Could you check a few things on this model? Use its own coordinates, in mm. A direction names the side the tool comes from. Give positions to 0.01 mm unless a question says otherwise; leave off trailing zeros. Loops run counter-clockwise (first coordinate to the right, second up) from the corner with the lowest first, then second, coordinate; pieces in that order, holes last. Notation, with made-up numbers: M 72,42 L 82,42 A17 cw 82,49 Z; hole C -10.5,61.5 d11. An arc over 180 degrees is marked long. Answer in a Markdown table with one row per item. Add a question column.
1. If we section it at C-C on z = 10: List the corners of the cut face in (x, y) for me.
2. If we section it at D-D on y = -9: List the corners of the cut face in (x, z) for me (3 decimals), then the cut area to 3 significant figures.
3. I'm going to push flat-ended pins straight in: pin 1 Ø3.5 at (y, z) = (7, 10) entering from +X; pin 2 Ø1 at (y, z) = (-5, 1) entering from -X; pin 3 Ø1.8 at (x, z) = (-8.5, 10.5) entering from -Y; pin 4 Ø5 at (x, y) = (-8.5, -8.5) entering from +Z. Where does each tip first touch, or does it pass through?
4. Which directions (+Z, -Z, +X, -X, +Y, -Y) give clear straight access to the entire face, cutting with the end or side of a thin tool? Please do faces 4 (the flat face through (-6, 6, 8)), 5 (the cylindrical face through (-6.57, 6.52, 2.45)), 6 (the cylindrical face through (-9.993, 6.599, 7.752)).
5. I need wall thicknesses on line 1 along Y through (x, z) = (0, 0.5) (3 decimals); line 2 along Z through (x, y) = (-7.05, 6.5); line 3 along Z through (x, y) = (-3.75, 0). Which ranges of each line are inside material? Lowest first, please. Write a range as from..to.
6. If we section it at A-A on y = 6.5: List the corners of the cut face in (x, z) for me, then the cut area to 3 significant figures.
7. If we section it at B-B on x = 0: List the corners of the cut face in (y, z) for me (3 decimals), then the cut area to 3 significant figures.
8. Thinking about a two-plate mould opening in Y: for faces 1 (the cylindrical face through (-0.179, -7.637, 1.014)), 2 (the flat face through (-4.5, -6, 1)), 3 (the cylindrical face through (-4.95, 1.57, 1.06)), which applies, released by +Y, released by -Y, zero draft, split by the parting line, or undercut?
```python
from build123d import *

# Parameters (mm, degrees)
SKETCH1_W           = 9
SKETCH1_H           = 22
BOSS_EXTRUDE1_DEPTH = 2
SKETCH2_R           = 2.5
SKETCH2_R_2         = 1.375
CUT_EXTRUDE1_DEPTH  = 2
SKETCH3_W           = 2
SKETCH3_H           = 9
BOSS_EXTRUDE2_DEPTH = 5
SKETCH5_W           = 2.5
SKETCH5_H           = 9
BOSS_EXTRUDE4_DEPTH = 12.5
SKETCH6_R           = 1.75
CUT_EXTRUDE2_DEPTH  = 2.5
SKETCH7_R           = 2.25
BOSS_EXTRUDE5_DEPTH = 1
SKETCH8_R           = 1.75
CUT_EXTRUDE3_DEPTH  = 1
SKETCH9_R           = 2.25
BOSS_EXTRUDE6_DEPTH = 1
SKETCH10_R          = 1.75
CUT_EXTRUDE4_DEPTH  = 1
FILLET1_R           = 1.5
FILLET2_R           = 1.5
SKETCH11_W          = 9
SKETCH11_H          = 2
BOSS_EXTRUDE7_DEPTH = 1.5


with BuildPart() as part:
    # Sketch1 → Boss-Extrude1 (new body)
    with BuildSketch(Plane.XY):
        Rectangle(SKETCH1_W, SKETCH1_H)
    extrude(amount=BOSS_EXTRUDE1_DEPTH)

    # Sketch2 → Cut-Extrude1 (cut)
    with BuildSketch(Plane.XY.offset(2)):
        with Locations((0, 6.5)):
            Circle(SKETCH2_R)
        with Locations((0, -9)):
            Circle(SKETCH2_R_2)
    extrude(amount=-CUT_EXTRUDE1_DEPTH, mode=Mode.SUBTRACT)

    # Sketch3 → Boss-Extrude2 (add)
    with BuildSketch(Plane.ZY.offset(4.5)):
        with Locations((1, 6.5)):
            Rectangle(SKETCH3_W, SKETCH3_H)
    extrude(amount=BOSS_EXTRUDE2_DEPTH)

    # Sketch5 → Boss-Extrude4 (add)
    with BuildSketch(Plane.XY.offset(2)):
        with Locations((-8.25, 6.5)):
            Rectangle(SKETCH5_W, SKETCH5_H)
    extrude(amount=BOSS_EXTRUDE4_DEPTH)

    # Sketch6 → Cut-Extrude2 (cut)
    with BuildSketch(Plane(origin=(-7, 0, 0), x_dir=(0, 0, -1), z_dir=(1, 0, 0))):
        with Locations((-10, 6.5)):
            Circle(SKETCH6_R)
    extrude(amount=-CUT_EXTRUDE2_DEPTH, mode=Mode.SUBTRACT)

    # Sketch7 → Boss-Extrude5 (add)
    with BuildSketch(Plane(origin=(-7, 0, 0), x_dir=(0, 0, -1), z_dir=(1, 0, 0))):
        with Locations((-10, 6.5)):
            Circle(SKETCH7_R)
    extrude(amount=BOSS_EXTRUDE5_DEPTH)

    # Sketch8 → Cut-Extrude3 (cut)
    with BuildSketch(Plane(origin=(-6, 0, 0), x_dir=(0, 0, -1), z_dir=(1, 0, 0))):
        with Locations((-10, 6.5)):
            Circle(SKETCH8_R)
    extrude(amount=-CUT_EXTRUDE3_DEPTH, mode=Mode.SUBTRACT)

    # Sketch9 → Boss-Extrude6 (add)
    with BuildSketch(Plane.ZY.offset(9.5)):
        with Locations((10, 6.5)):
            Circle(SKETCH9_R)
    extrude(amount=BOSS_EXTRUDE6_DEPTH)

    # Sketch10 → Cut-Extrude4 (cut)
    with BuildSketch(Plane.ZY.offset(10.5)):
        with Locations((10, 6.5)):
            Circle(SKETCH10_R)
    extrude(amount=-CUT_EXTRUDE4_DEPTH, mode=Mode.SUBTRACT)

    # Fillet1
    fillet1_edges = [part.edges().sort_by_distance(p)[0] for p in [
        (-7, 6.5, 2),
    ]]
    fillet(fillet1_edges, radius=FILLET1_R)

    # Fillet2
    fillet2_edges = [part.edges().sort_by_distance(p)[0] for p in [
        (-4.5, 2, 1),
    ]]
    fillet(fillet2_edges, radius=FILLET2_R)

    # Sketch11 → Boss-Extrude7 (add)
    with BuildSketch(Plane.XZ.offset(11)):
        with Locations((0, 1)):
            Rectangle(SKETCH11_W, SKETCH11_H)
    extrude(amount=BOSS_EXTRUDE7_DEPTH)


solid = part.part
```
Results:
| question | item | result |
|---|---|---|
| 1 | outline | M -10.5,4.25 L -9.5,4.25 L -9.5,2 L -7,2 L -7,4.25 L -6,4.25 L -6,4.75 L -10.5,4.75 Z; M -10.5,8.25 L -6,8.25 L -6,8.75 L -7,8.75 L -7,11 L -9.5,11 L -9.5,8.75 L -10.5,8.75 Z |
| 2 | outline | M -4.5,0 L -1.375,0 L -1.375,2 L -4.5,2 Z; M 1.375,0 L 4.5,0 L 4.5,2 L 1.375,2 Z |
| 2 | area | 12.5 mm2 |
| 3 | pin 1 | x = -6 |
| 3 | pin 2 | x = -4.5 |
| 3 | pin 3 | y = 2 |
| 3 | pin 4 | through |
| 4 | face 4 | +Z, +X, +Y, -Y |
| 4 | face 5 | +X, +Y, -Y |
| 4 | face 6 | -X |
| 5 | line 1 | -12.5..-10.375, -7.625..4, 9..11 |
| 5 | line 2 | 0..8.25, 11.75..14.5 |
| 5 | line 3 | 0..2 |
| 6 | outline | M -10.5,7.75 L -9.5,7.75 L -9.5,0 L -2.5,0 L -2.5,2 L -5.5,2 A1.5 cw -7,3.5 L -7,7.75 L -6,7.75 L -6,8.25 L -10.5,8.25 Z; M -10.5,11.75 L -6,11.75 L -6,12.25 L -7,12.25 L -7,14.5 L -9.5,14.5 L -9.5,12.25 L -10.5,12.25 Z; M 2.5,0 L 4.5,0 L 4.5,2 L 2.5,2 Z |
| 6 | area | 43.0 mm2 |
| 7 | outline | M -12.5,0 L -10.375,0 L -10.375,2 L -12.5,2 Z; M -7.625,0 L 4,0 L 4,2 L -7.625,2 Z; M 9,0 L 11,0 L 11,2 L 9,2 Z |
| 7 | area | 31.5 mm2 |
| 8 | face 1 | undercut |
| 8 | face 2 | zero draft |
| 8 | face 3 | released by -Y |
